For this review, take the finished solid that the model builds, in its own axes (mm). Face numbers are marked on the shaded views. A direction names the side the tool comes from. Round coordinates to 2 decimals unless told otherwise and drop trailing zeros. Loops run counter-clockwise (first coordinate to the right, second up) from the corner with the lowest first, then second, coordinate; pieces in that order, holes last.
1. To check wall thickness, follow line 1 along Y through (x, z) = (-56, -121.5); line 2 along X through (y, z) = (-21.5, -115); line 3 along Z through (x, y) = (26.5, -20). State the ranges of each line that lie inside material, in increasing order.
2. Clearance check with flat-ended pins moving along their axes: pin 1 Ø1 at (x, y) = (-37.5, -18.5) entering from +Z; pin 2 Ø2 at (x, z) = (35.5, -79.5) entering from +Y; pin 3 Ø2 at (y, z) = (20.5, -188.5) entering from -X. State where each tip first meets the part, or that it passes through.
3. Consider section A-A on x = -9.5. State the section outline as (y, z) points, then the cut area to 3 significant figures.
4. Tool access review of the marked faces 1, 2 and 3: name each direction out of +Z, -Z, +X, -X, +Y, -Y from which nothing blocks a thin tool from reaching the whole face with its end or side.
5. Consider section B-B on z = -92.5. State the section outline as (x, y) points, then the cut area to 3 significant figures.
6. Draft analysis for pull direction X (two halves, no side actions). For the marked faces 4, 5 and 6, state which applies: released by +X, released by -X, zero draft, split by the parting line, or undercut.
7. Consider section C-C on x = -32.5. State the section outline as (y, z) points.
from build123d import *

# Parameters (mm, degrees)
SKETCH1_R               = 45
BOSS_EXTRUDE1_DEPTH     = 35
CUT_EXTRUDE1_DEPTH      = 30
BOSS_EXTRUDE6_START     = 30
SKETCH4_R               = 22.5
SKETCH4_R_2             = 45
BOSS_EXTRUDE6_DEPTH     = 30
CUT_EXTRUDE5_DEPTH      = 233.326481949
CUT_EXTRUDE5_DEPTH_BACK = 233.326481949
SKETCH11_R              = 17.5
FILLET5_R               = 10
FILLET7_R               = 5
FILLET8_R               = 5


with BuildPart() as part:
    # Sketch1 → Boss-Extrude1 (new body)
    with BuildSketch(Plane(origin=(0, 0, 0), x_dir=(1, 0, 0), z_dir=(0, 1, 0))):
        Polygon((46.859255168, 63.80155033), (-83.545615043, 63.80155033), (-97.357476794, 66.23695421), (-86.281022646, 129.054647247), (-78.894964498, 127.752285914), (-74.254340533, 154.070572239), (0, 208.019508525), (75.819867549, 152.933150283), align=None)
        with Locations(Location((0, 127.60310066, 0), (0, 0, 90))):
            Circle(SKETCH1_R, mode=Mode.SUBTRACT)
    extrude(amount=BOSS_EXTRUDE1_DEPTH)

    # Sketch2 → Cut-Extrude1 (cut)
    with BuildSketch(Plane(origin=(0, 35, 0), x_dir=(1, 0, 0), z_dir=(0, 1, 0))):
        Polygon((69.942015026, 151.023320226), (0, 201.839168637), (-69.681093857, 151.212890552), (-74.839166621, 121.960006261), (-82.225224769, 123.262367593), (-91.56519714, 70.292752087), (-83.108171726, 68.80155033), (43.226542528, 68.80155033), align=None)
    extrude(amount=-CUT_EXTRUDE1_DEPTH, mode=Mode.SUBTRACT)

    # Sketch4 → Boss-Extrude6 (add)
    with BuildSketch(Plane.XZ.offset(BOSS_EXTRUDE6_START)):
        with BuildLine():
            ThreePointArc((-38.294135291, -80.643268154), (-86.152709956, -81.952683716), (-60.360710902, -122.287910539))
            ThreePointArc((-60.360710902, -122.287910539), (-53.229459059, -124.750444519), (-49.848314613, -131.494826529))
            ThreePointArc((-49.848314613, -131.494826529), (44.180876901, -151.013570888), (-24.772660509, -84.171369273))
            ThreePointArc((-24.772660509, -84.171369273), (-32.2519207, -85.161062892), (-38.294135291, -80.643268154))
        make_face()
        with Locations(Location((-61.853227661, -94.828442341, 0), (0, 0, 270))):
            Circle(SKETCH4_R, mode=Mode.SUBTRACT)
        with Locations(Location((0, -127.60310066, 0), (0, 0, 270))):
            Circle(SKETCH4_R_2, mode=Mode.SUBTRACT)
    extrude(amount=-BOSS_EXTRUDE6_DEPTH)

    # Sketch11 → Cut-Extrude5 (cut, two sides: drawn at the far end of the back side and taken through both)
    with BuildSketch(Plane.XZ.offset(-CUT_EXTRUDE5_DEPTH_BACK)):
        with Locations(Location((-61.853227661, -94.828442341, 0), (0, 0, 270))):
            Circle(SKETCH11_R)
    extrude(amount=CUT_EXTRUDE5_DEPTH + CUT_EXTRUDE5_DEPTH_BACK, mode=Mode.SUBTRACT)

    # Fillet5
    fillet5_edges = [part.edges().sort_by_distance(p)[0] for p in [
        (-97.357476794, 17.5, -66.23695421),
        (-74.254340533, 17.5, -154.070572239),
        (0, 17.5, -208.019508525),
        (75.819867549, 17.5, -152.933150283),
        (46.859255168, 17.5, -63.80155033),
    ]]
    fillet(fillet5_edges, radius=FILLET5_R)

    # Fillet7
    fillet7_edges = [part.edges().sort_by_distance(p)[0] for p in [
        (-78.894964498, 17.5, -127.752285914),
    ]]
    fillet(fillet7_edges, radius=FILLET7_R)

    # Fillet8
    fillet8_edges = [part.edges().sort_by_distance(p)[0] for p in [
        (-86.281022646, 17.5, -129.054647247),
    ]]
    fillet(fillet8_edges, radius=FILLET8_R)


solid = part.part
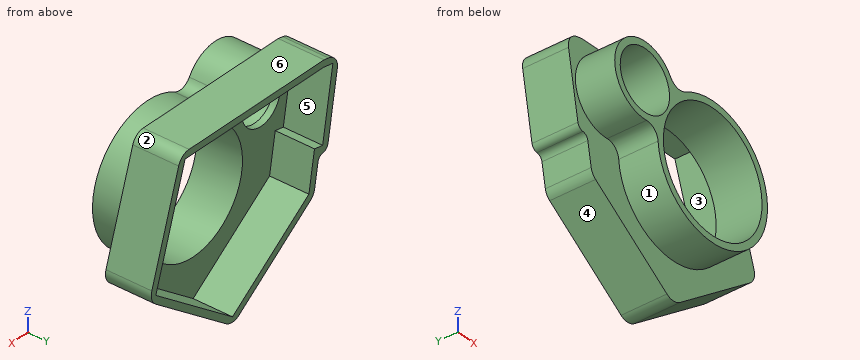
Resolved:
1. line 1: y = -30 to 5
1. line 2: x = -80.54 to -71.82, -51.89 to -43.2, 43.2 to 48.39
1. line 3: z = -170 to -163.97, -91.23 to -85.2
2. pin 1: stops at z = -81.1
2. pin 2: stops at y = 5
2. pin 3: stops at x = -28.24
3. outline: (-30, -176.69) - (0, -176.69) - (0, -201.12) - (35, -201.12) - (35, -194.94) - (5, -194.94) - (5, -171.59) - (-30, -171.59) - close; (-30, -83.62) - (5, -83.62) - (5, -68.8) - (35, -68.8) - (35, -63.8) - (0, -63.8) - (0, -78.51) - (-30, -78.51) - close
3. area: 888 mm2
4. face 1: -Y
4. face 2: +Z, +X, +Y, -Y
4. face 3: +Y
5. outline: (-92.73, 0) - (-89.25, 0) - (-89.25, -30) - (-84.23, -30) - (-84.23, 0) - (-79.2, 0) - (-79.2, 5) - (-87.65, 5) - (-87.65, 35) - (-92.73, 35) - close; (-44.51, 0) - (-39.47, 0) - (-39.47, -30) - (-28.16, -30) - (-28.16, 5) - (-44.51, 5) - close; (28.16, -30) - (35.61, -30) - (35.61, 0) - (56.18, 0) - (56.18, 35) - (50.93, 35) - (50.93, 5) - (28.16, 5) - close
5. area: 1,310 mm2
6. face 4: released by -X
6. face 5: undercut
6. face 6: zero draft
7. outline: (-30, -165.6) - (0, -165.6) - (0, -184.41) - (35, -184.41) - (35, -178.23) - (5, -178.23) - (5, -158.73) - (-30, -158.73) - close; (-30, -96.48) - (5, -96.48) - (5, -68.8) - (35, -68.8) - (35, -63.8) - (0, -63.8) - (0, -85.09) - (-30, -85.09) - close
